from build123d import *

# Parameters (mm, degrees)
FILLET3_R = 1
FILLET4_R = 1


with BuildPart() as part:
    # Sketch1 → Revolve1 (revolve)
    with BuildSketch(Plane(origin=(0, 0, 0), x_dir=(1, 0, 0), z_dir=(0, 1, 0)), mode=Mode.PRIVATE) as revolve1_sk:
        Polygon((8.5, 30), (9.5, 0), (8.5, -30), (11, -30), (12, 0), (11, 30), align=None)
    revolve(revolve1_sk.sketch.rotate(Axis((0, 0, -39.2734375), (0, 0, 1)), 180), axis=Axis((0, 0, -39.2734375), (0, 0, 1)))

    # Fillet3
    fillet3_edges = [part.edges().sort_by_distance(p)[0] for p in [
        (11, 0, -30),
        (12, 0, 0),
        (11, 0, 30),
        (8.5, 0, 30),
        (8.5, 0, -30),
    ]]
    fillet(fillet3_edges, radius=FILLET3_R)

    # Fillet4
    # the kernel refuses this fillet: 1 mm, written as the material it adds along each edge
    with BuildSketch(Plane(origin=(0, 0, 0), x_dir=(-1, 0, 0), z_dir=(0, 1, 0))) as fillet4_piece_1:
        with BuildLine():
            CenterArc((9.5 - FILLET4_R * 1.00055540132, 0), FILLET4_R, 358.090847567, 3.818304866)
            Line((9.5 - FILLET4_R * 0.00111049434109, FILLET4_R * 0.0333148302326), (9.5, 0))
            Line((9.5, 0), (9.5 - FILLET4_R * 0.00111049434109, -FILLET4_R * 0.0333148302326))
        make_face()
    revolve(axis=Axis((0, 0, 0), (0, 0, 1)))


solid = part.part
Here's how the part is built. I have some questions about the finished solid (model axes, mm). A direction names the side the tool comes from. Round coordinates to 2 decimals unless told otherwise and drop trailing zeros. Loops run counter-clockwise (first coordinate to the right, second up) from the corner with the lowest first, then second, coordinate; pieces in that order, holes last. Notation, with made-up numbers: M 54,68.25 L 82,68.25 A21 cw 82,94.25 Z; hole C 4.5,-38.75 d6. An arc over 180 degrees is marked long. Write each question's results on one line, items separated by ' | '. Start each with the question number.
(1) If I drill on probe 1 along X at (y, z) = (-4.25, -19); probe 2 along X at (y, z) = (-6.5, -21.5); probe 3 along Y at (x, z) = (3.5, -4), over which ranges is the centre line in solid material (lowest first)? Write a range as from..to.
(2) Will these pins go through, and if not, where does the flat tip stop? P1, Ø10, axis at y = -5, z = 15.5, coming from the +X side; P2, Ø5, axis at y = -0.5, z = 23.5, coming from the +X side; P3, Ø1.5, axis at x = -9.5, z = 16.5, coming from the -Y side.
(3) I want a section at A-A (x = 0). Please give me the cut outline in (y, z), then the cut area to 3 significant figures.
(4) I want a section at D-D (z = -10). Please give me the cut outline in (x, y), then the cut area to 3 significant figures.
(5) Thinking about a two-plate mould opening in X: for faces 1 (the conical face through (-8.607, -2.71, -14.297)), 2 (the flat face through (4, 9, 30)), 3 (the conical face through (2.5, 11.25, 14.31)), which applies, pulls with the +X half, pulls with the -X half, needs draft (parallel to the pull), parting line crosses it, or undercut?
(6) On a 3-axis mill with a long thin cutter (end or side, diameter ignored), from which of +Z, -Z, +X, -X, +Y, -Y can I reach the whole of each face in a straight line? I mean faces 4 (the conical face through (2.495, 11.236, -14.72)), 5 (the conical face through (1.953, 8.796, 14.703)), 6 (the flat face through (-4, 9, -30)). Say none if no direction works.
(7) I want a section at C-C (z = -4). Please give me the cut outline in (x, y).
Solved:
1) probe 1: x = -10.54..-7.78, 7.78..10.54 | probe 2: x = -9.22..-5.91, 5.91..9.22 | probe 3: y = -11.34..-8.69, 8.69..11.34
2) P1: stops at x = 11.55 | P2: stops at x = 11.3 | P3: stops at y = -7.39
3) outline: M -12,0 L -11.03,-29.03 A1 ccw -10.03,-30 L -9.53,-30 A1 ccw -8.53,-28.97 L -9.5,-0.03 A1 cw -9.5,0.03 L -8.53,28.97 A1 ccw -9.53,30 L -10.03,30 A1 ccw -11.03,29.03 Z; M 8.53,-28.97 A1 ccw 9.53,-30 L 10.03,-30 A1 ccw 11.03,-29.03 L 12,0 L 11.03,29.03 A1 ccw 10.03,30 L 9.53,30 A1 ccw 8.53,28.97 L 9.5,0.03 A1 cw 9.5,-0.03 Z | area: 298 mm²
4) outline: C 0,0 d23.33; hole C 0,0 d18.33 | area: 164 mm²
5) face 1: undercut | face 2: needs draft | face 3: parting line crosses it
6) face 4: -Z | face 5: none | face 6: -Z, +X, -X, +Y, -Y
7) outline: C 0,0 d23.73; hole C 0,0 d18.73
